from build123d import *

# Parameters (mm, degrees)
ESQUISSE1_W                          = 300
ESQUISSE1_H                          = 240
BOSS_EXTRU_1_DEPTH                   = 5
TENON_START                          = -190
TENON_ET_MORTAISE_TENON1_OUTLINE_W   = 5
TENON_ET_MORTAISE_TENON1_OUTLINE_H   = 5
TENON_ET_MORTAISE_TENON1_DEPTH       = 42
TENON_START_2                        = -82
TENON_ET_MORTAISE_TENON1_2_OUTLINE_W = 5
TENON_ET_MORTAISE_TENON1_2_OUTLINE_H = 5
TENON_ET_MORTAISE_TENON1_2_DEPTH     = 42
TENON_ET_MORTAISE_TENON2_OUTLINE_W   = 5
TENON_ET_MORTAISE_TENON2_OUTLINE_H   = 5
TENON_ET_MORTAISE_TENON2_DEPTH       = 42
TENON_ET_MORTAISE_TENON2_2_OUTLINE_W = 5
TENON_ET_MORTAISE_TENON2_2_OUTLINE_H = 5
TENON_ET_MORTAISE_TENON2_2_DEPTH     = 42
ESQUISSE2_R                          = 5.05
ENL_V_MAT_EXTRU_1_DEPTH              = 10
ESQUISSE3_W                          = 100
ESQUISSE3_H                          = 46
ENL_V_MAT_EXTRU_3_DEPTH              = 10
ESQUISSE5_R                          = 1.5
ENL_V_MAT_EXTRU_4_DEPTH              = 10


# Read off the part's stored shape, not the designer's step: Tenon et mortaise-Tenon1, Tenon et mortaise-Tenon2
with BuildPart() as part:
    # Esquisse1 → Boss.-Extru.1 (new body)
    with BuildSketch(Plane.XY):
        with Locations((-150, -120)):
            Rectangle(ESQUISSE1_W, ESQUISSE1_H)
    extrude(amount=BOSS_EXTRU_1_DEPTH)

    # Tenon et mortaise-Tenon1 outline → Tenon et mortaise-Tenon1 (add)
    with BuildSketch(Plane(origin=(0, 0, 0), x_dir=(1, 0, 0), z_dir=(0, 1, 0)).offset(TENON_START)):
        with Locations((-302.5, -2.5)):
            Rectangle(TENON_ET_MORTAISE_TENON1_OUTLINE_W, TENON_ET_MORTAISE_TENON1_OUTLINE_H)
    extrude(amount=TENON_ET_MORTAISE_TENON1_DEPTH)

    # Tenon et mortaise-Tenon1 2 outline → Tenon et mortaise-Tenon1 2 (add)
    with BuildSketch(Plane(origin=(0, 0, 0), x_dir=(1, 0, 0), z_dir=(0, 1, 0)).offset(TENON_START_2)):
        with Locations((-302.5, -2.5)):
            Rectangle(TENON_ET_MORTAISE_TENON1_2_OUTLINE_W, TENON_ET_MORTAISE_TENON1_2_OUTLINE_H)
    extrude(amount=TENON_ET_MORTAISE_TENON1_2_DEPTH)

    # Tenon et mortaise-Tenon2 outline → Tenon et mortaise-Tenon2 (add)
    with BuildSketch(Plane(origin=(0, 0, 0), x_dir=(1, 0, 0), z_dir=(0, 1, 0)).offset(TENON_START)):
        with Locations((2.5, -2.5)):
            Rectangle(TENON_ET_MORTAISE_TENON2_OUTLINE_W, TENON_ET_MORTAISE_TENON2_OUTLINE_H)
    extrude(amount=TENON_ET_MORTAISE_TENON2_DEPTH)

    # Tenon et mortaise-Tenon2 2 outline → Tenon et mortaise-Tenon2 2 (add)
    with BuildSketch(Plane(origin=(0, 0, 0), x_dir=(1, 0, 0), z_dir=(0, 1, 0)).offset(TENON_START_2)):
        with Locations((2.5, -2.5)):
            Rectangle(TENON_ET_MORTAISE_TENON2_2_OUTLINE_W, TENON_ET_MORTAISE_TENON2_2_OUTLINE_H)
    extrude(amount=TENON_ET_MORTAISE_TENON2_2_DEPTH)

    # Esquisse2 → Enlèv. mat.-Extru.1 (cut)
    with BuildSketch(Plane.XY.offset(5)):
        with Locations((-231.788943558, -89.854265633)):
            Circle(ESQUISSE2_R)
        with Locations((-146.505843122, -89.854265633)):
            Circle(ESQUISSE2_R)
        with Locations((-59.877583373, -89.854265633)):
            Circle(ESQUISSE2_R)
    extrude(amount=-ENL_V_MAT_EXTRU_1_DEPTH, mode=Mode.SUBTRACT)

    # Esquisse3 → Enlèv. mat.-Extru.3 (cut)
    with BuildSketch(Plane.XY.offset(5)):
        with Locations((-148.865660617, -38.407404502)):
            Rectangle(ESQUISSE3_W, ESQUISSE3_H)
    extrude(amount=-ENL_V_MAT_EXTRU_3_DEPTH, mode=Mode.SUBTRACT)

    # Esquisse5 → Enlèv. mat.-Extru.4 (cut)
    with BuildSketch(Plane.XY.offset(5)):
        with Locations((-102.365660617, -10.407404502)):
            Circle(ESQUISSE5_R)
        with Locations((-195.365660617, -10.407404502)):
            Circle(ESQUISSE5_R)
        with Locations((-195.365660617, -65.407404502)):
            Circle(ESQUISSE5_R)
        with Locations((-102.365660617, -65.407404502)):
            Circle(ESQUISSE5_R)
    extrude(amount=-ENL_V_MAT_EXTRU_4_DEPTH, mode=Mode.SUBTRACT)


solid = part.part
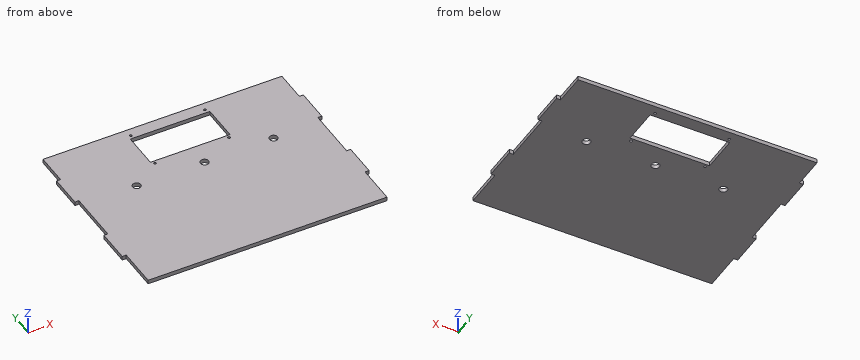
Can you work these out from the model? Positions are in its coordinate system, mm. Coordinates: 2 decimals unless noted, no trailing zeros. Loops run counter-clockwise (first coordinate to the right, second up) from the corner with the lowest first, then second, coordinate; pieces in that order, holes last. Notation, with made-up numbers: M 63.5,84 L 101.5,84 A12 ccw 101.5,100 Z; hole C -16.5,-17.5 d1. An arc over 180 degrees is marked long. Return JSON: item names as keys, results as strings. Group by question number.
Item 1: I'm going to push flat-ended pins straight in: pin 1 Ø1.5 at (x, z) = (-303.5, 3.5) entering from +Y; pin 2 Ø2.5 at (y, z) = (-12, 1.5) entering from -X; pin 3 Ø2.5 at (y, z) = (-215.5, 2) entering from +X. Where does each tip first touch, or does it pass through?
Item 2: Imagine slicing it at D-D (y = -217). Please give me the cut outline in (x, z), and give its area (3 significant figures).
Item 3: If I drill on L1, parallel to X at y = -57, z = 2.85; L2, parallel to Y at x = -177.5, z = 1.3; L3, parallel to X at y = -66, z = 4.7, over which ranges is the centre line in solid material (lowest first)? Write a range as from..to.
Item 4: Imagine slicing it at B-B (x = -116.5). Please give me the cut outline in (y, z).
Item 5: Imagine slicing it at A-A (y = -57). Please give me the cut outline in (x, z).
Item 6: Imagine slicing it at C-C (z = 1.65). Give the number of separate pieces and of enclosed holes in the cut face, and give its area (3 significant figures).
Verdict:
{
 "1": {"pin 1": "stops at y = -40", "pin 2": "stops at x = -300", "pin 3": "stops at x = 0"},
 "2": {"outline": "M -300,0 L 0,0 L 0,5 L -300,5 Z", "area": "1,500 mm^2"},
 "3": {"L1": "x = -305..-198.87, -98.87..5", "L2": "y = -240..-61.41, -15.41..0", "L3": "x = -305..-196.74, -193.99..-103.74, -100.99..5"},
 "4": {"outline": "M -240,0 L -61.41,0 L -61.41,5 L -240,5 Z; M -15.41,0 L 0,0 L 0,5 L -15.41,5 Z"},
 "5": {"outline": "M -305,0 L -198.87,0 L -198.87,5 L -305,5 Z; M -98.87,0 L 5,0 L 5,5 L -98.87,5 Z"},
 "6": {"separate pieces": "1", "enclosed holes": "8", "area": "68,000 mm^2"}
}
